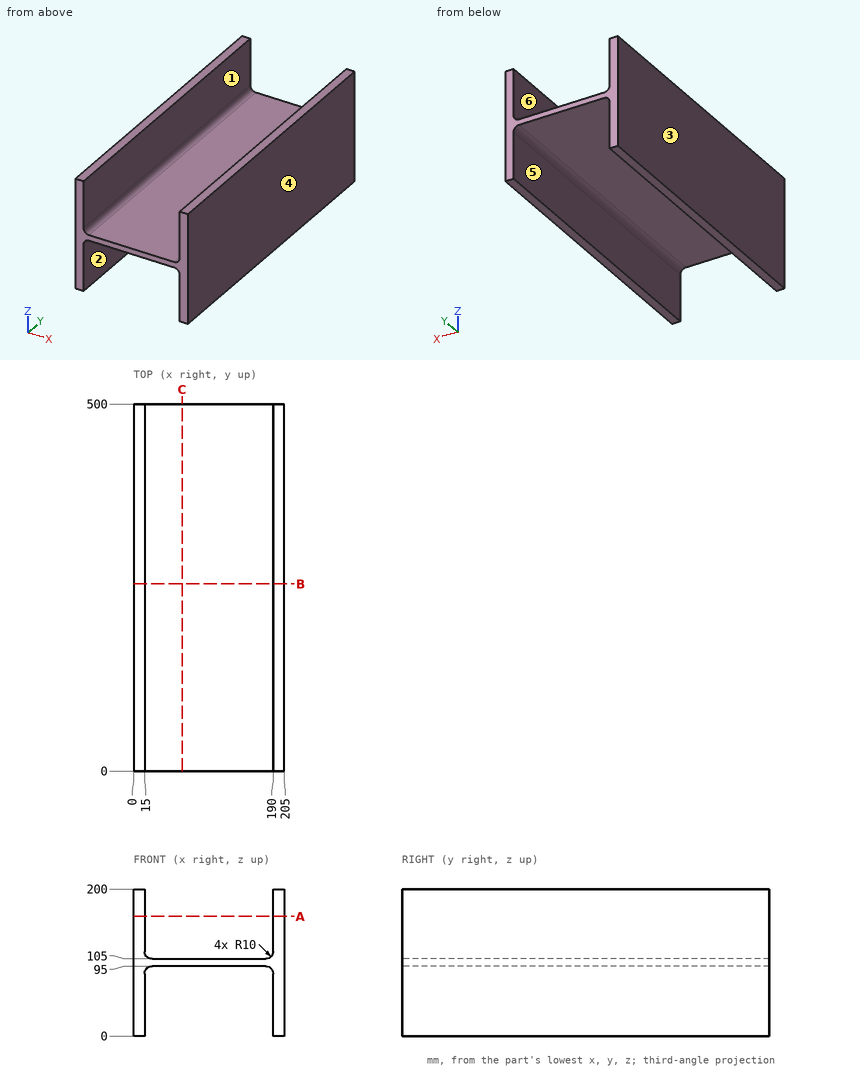
Input: dimensioned drawing with shaded views. Units: mm. Origin: part minimum x, y, z. A direction names the side the tool comes from. Round coordinates to 2 decimals unless told otherwise and drop trailing zeros. Order: outer loops, then holes, each group sorted by start corner. A loop starts at its lowest first (then second) coordinate and runs counter-clockwise, first axis right, second up. Notation, with made-up numbers: M -15,37.5 L -6,37.5 A20 cw -6,73.5 Z; hole C -28,85.25 d5. An arc over 180 degrees is marked long. Use one line per item in the form item = value. Start each with the question number.
Q1. Mould query, pull axis X, two halves, no side actions, for the marked faces 1, 2, 3 and 4. Classes: +X half, -X half, draft (parallel to the pull), parting line (faces both ways), or undercut.
Q2. Pin query (flat end, axial travel): pin 1 Ø6 at (x, y) = (152, 404) entering from -Z; pin 2 Ø2 at (y, z) = (285, 70) entering from -X; pin 3 Ø6 at (x, y) = (180, 356.5) entering from +Z. Return the tip coordinate at first contact, or that it passes through.
Q3. Cut plane C-C (x = 66). Return loops of the section in (y, z).
Q4. Cut plane A-A (z = 163). Return loops of the section in (x, y).
Q5. Material intervals for line 1 (X direction, y = 144, z = 166); line 2 (Z direction, x = 102, y = 378.5); line 3 (X direction, y = 63.5, z = 91.5), sorted ascending. Write a range as [from, to].
Q6. Cut plane B-B (y = 255). Return loops of the section in (x, z).
Q7. Access query for the marked faces 5 and 6. Directions: +Z, -Z, +X, -X, +Y, -Y. A direction counts if a zero-diameter tool reaches every point of the face in a straight line with its end or side. Return the directions, or none.
Geometry results:
q1.face_1 = undercut
q1.face_2 = undercut
q1.face_3 = -X half
q1.face_4 = +X half
q2.pin_1 = 95
q2.pin_2 = 0
q2.pin_3 = 105.46
q3.outline = M 0,95 L 500,95 L 500,105 L 0,105 Z
q4.outline = M 0,0 L 15,0 L 15,500 L 0,500 Z; M 190,0 L 205,0 L 205,500 L 190,500 Z
q5.line_1 = [0, 15], [190, 205]
q5.line_2 = [95, 105]
q5.line_3 = [0, 17.4], [187.6, 205]
q6.outline = M 0,0 L 15,0 L 15,85 A10 cw 25,95 L 180,95 A10 cw 190,85 L 190,0 L 205,0 L 205,200 L 190,200 L 190,115 A10 cw 180,105 L 25,105 A10 cw 15,115 L 15,200 L 0,200 Z
q7.face_5 = -Z, +Y, -Y
q7.face_6 = +Z, +Y, -Y
